```python
from build123d import *

# Parameters (mm, degrees)
EXTRUDE_3_DEPTH     = 5
SKETCH_2_6_W        = 56
SKETCH_2_6_H        = 60
EXTRUDE_4_DEPTH     = 7
SKETCH_4_W          = 56
SKETCH_4_H          = 60
EXTRUDE_5_DEPTH     = 5
EXTRUDE_6_DEPTH     = 19
SKETCH_7_W          = 13
SKETCH_7_H          = 15
CUT_EXTRUDE_1_DEPTH = 34


with BuildPart() as part:
    # Эскиз2 → Бобышка-Вытянуть3 (new body)
    with BuildSketch(Plane(origin=(0, 0, 0), x_dir=(1, 0, 0), z_dir=(0, 1, 0))):
        Polygon((0, 0), (150, 0), (150, 70), (0, 70), (0, 5), align=None)
    extrude(amount=EXTRUDE_3_DEPTH)

    # Эскиз2<6> → Бобышка-Вытянуть4 (add)
    with BuildSketch(Plane(origin=(0, 0, 0), x_dir=(1, 0, 0), z_dir=(0, 1, 0))):
        Polygon((0, 0), (150, 0), (150, 70), (0, 70), (0, 5), align=None)
        with Locations((31, 35)):
            Rectangle(SKETCH_2_6_W, SKETCH_2_6_H, mode=Mode.SUBTRACT)
    extrude(amount=EXTRUDE_4_DEPTH)

    # Эскиз4 → Бобышка-Вытянуть5 (add)
    with BuildSketch(Plane(origin=(0, 5, 0), x_dir=(1, 0, 0), z_dir=(0, 1, 0))):
        with Locations((31, 35)):
            Rectangle(SKETCH_4_W, SKETCH_4_H)
    extrude(amount=-EXTRUDE_5_DEPTH)

    # Эскиз5 → Бобышка-Вытянуть6 (add)
    with BuildSketch(Plane(origin=(0, 7, 0), x_dir=(1, 0, 0), z_dir=(0, 1, 0))):
        Polygon((84, 52), (69, 52), (67, 52), (67, 18), (84, 18), align=None)
        Polygon((69, 23), (69, 35), (69, 47), (82, 47), (82, 35), (82, 23), align=None, mode=Mode.SUBTRACT)
    extrude(amount=EXTRUDE_6_DEPTH)

    # Эскиз7 → Вырез-Вытянуть1 (cut)
    with BuildSketch(Plane.XY.offset(-18)):
        with Locations((75.5, 14.5)):
            Rectangle(SKETCH_7_W, SKETCH_7_H)
    extrude(amount=-CUT_EXTRUDE_1_DEPTH, mode=Mode.SUBTRACT)


solid = part.part
```
Here's how the part is built. I have some questions about the finished solid (model axes, mm). A direction names the side the tool comes from. Coordinates: 2 decimals unless noted, no trailing zeros. Loops run counter-clockwise (first coordinate to the right, second up) from the corner with the lowest first, then second, coordinate; pieces in that order, holes last. Notation, with made-up numbers: (70.25, 80) - (97.25, 80) arc R24 cw to (97.25, 97) - close; hole circle Ø1 at (72, 77.25). An arc over 180 degrees is marked (long way). Return JSON: item names as keys, results as strings. Group by question number.
Item 1: If we section it at C-C on z = -39: Write out the boundary of the cut face in (x, y), and give its area (3 significant figures).
Item 2: I need wall thicknesses on line 1 (X direction, y = 17.5, z = -23); line 2 (Y direction, x = 91, z = -27); line 3 (Y direction, x = 37, z = -22). Which ranges of each line are inside material? Lowest first, please. Write a range as from..to.
Item 3: If we section it at B-B on x = 72.5: Write out the boundary of the cut face in (y, z).
Item 4: Will these pins go through, and if not, where does the flat tip stop? P1, Ø17, axis at x = 39, z = -37, coming from the +Y side; P2, Ø3, axis at x = 78, y = 23.5, coming from the +Z side; P3, Ø10, axis at y = 19.5, z = -13.5, coming from the -X side.
Item 5: If we section it at A-A on y = 12.75: Write out the boundary of the cut face in (x, z).
Item 6: If we section it at D-D on x = 17.5: Write out the boundary of the cut face in (y, z), and give its area (3 significant figures).
Item 7: On a 3-axis mill with a long thin cutter (end or side, diameter ignored), from which of +Z, -Z, +X, -X, +Y, -Y can I reach the whole of each face in a straight line? I mean faces 5 (the face through (75, 23, -18)), 6 (the face through (69, 16, -35)), 7 (the face through (76, 23, -52)). Say none if no direction works.
Item 8: We'd pull the mould along Y, two halves only. Please class faces 1 (the face through (76, 24, -23)), 2 (the face through (82, 16, -35)), 3 (the face through (31, 5, -35)), 4 (the face through (75, 22, -49)): +Y half, -Y half, draft (parallel to the pull), parting line (faces both ways), or undercut.
Calculated:
{
 "1": {"outline": "(0, 0) - (150, 0) - (150, 7) - (84, 7) - (84, 26) - (82, 26) - (82, 7) - (69, 7) - (69, 26) - (67, 26) - (67, 7) - (59, 7) - (59, 5) - (3, 5) - (3, 7) - (0, 7) - close", "area": "1,010 mm^2"},
 "2": {"line 1": "x = 67..69, 82..84", "line 2": "y = 0..7", "line 3": "y = 0..5"},
 "3": {"outline": "(0, -70) - (7, -70) - (7, 0) - (0, 0) - close; (22, -52) - (26, -52) - (26, -47) - (22, -47) - close; (22, -23) - (26, -23) - (26, -18) - (22, -18) - close"},
 "4": {"P1": "stops at y = 5", "P2": "stops at z = -18", "P3": "stops at x = 67"},
 "5": {"outline": "(67, -52) - (69, -52) - (69, -18) - (67, -18) - close; (82, -52) - (84, -52) - (84, -18) - (82, -18) - close"},
 "6": {"outline": "(0, -70) - (7, -70) - (7, -65) - (5, -65) - (5, -5) - (7, -5) - (7, 0) - (0, 0) - close", "area": "370 mm^2"},
 "7": {"face 5": "+Z, +X, -X, +Y", "face 6": "none", "face 7": "-Z, +X, -X, +Y"},
 "8": {"face 1": "draft", "face 2": "undercut", "face 3": "+Y half", "face 4": "undercut"}
}
